Geometry check sheet. Reference: drawing and pictorial views, mm from the part's lowest x, y, z. A direction names the side the tool comes from. Coordinates: 2 decimals unless noted, no trailing zeros. Loops run counter-clockwise (first coordinate to the right, second up) from the corner with the lowest first, then second, coordinate; pieces in that order, holes last. Notation, with made-up numbers: (53, 64.5) -> (91, 64.5) arc R22 cw to (91, 98.5) -> close; hole circle Ø6 at (43.5, -34). An arc over 180 degrees is marked (long way). Answer as a JSON object with one key per item and string values. Group by question number.
Q1. Set-up check for the marked faces 1 and 2: record each of +Z, -Z, +X, -X, +Y, -Y from which the full face is reachable in a straight line by a thin tool's end or side.
Q2. Cross-section at C-C on z = 7. Give the number of separate pieces and of enclosed holes in the cut face, and give its area (3 significant figures).
Q3. Cross-section at B-B on x = 40. Record the boundary of the cut face in (y, z), and give its area (3 significant figures).
Q4. Release check for a two-part mould opening along X. For the marked faces 3, 4 and 5 record: released by +X, released by -X, zero draft, split by the parting line, or undercut.
Q5. Cross-section at D-D on x = 15. Record the boundary of the cut face in (y, z) (1 decimal), and give its area (3 significant figures).
Q6. Gauge pin test, flat ends, axial feed: pin 1 Ø3 at (x, y) = (69.5, 45) entering from -Z; pin 2 Ø8 at (x, y) = (14.5, 39.5) entering from +Z; pin 3 Ø2.5 at (x, y) = (29.83, 12.39) entering from +Z; pin 4 Ø1 at (y, z) = (8, 2) entering from -X. Record the tip position at first contact, or that the pin passes through.
Q7. Cross-section at A-A on y = 40. Record the boundary of the cut face in (x, z).
Q8. Scan lines: L1, parallel to Y at x = 66.5, z = 2.75; L2, parallel to Y at x = 49, z = 6.75 (1 decimal); L3, parallel to Y at x = 12.5, z = 7.25. Record each from-to range of solid material in increasing order.
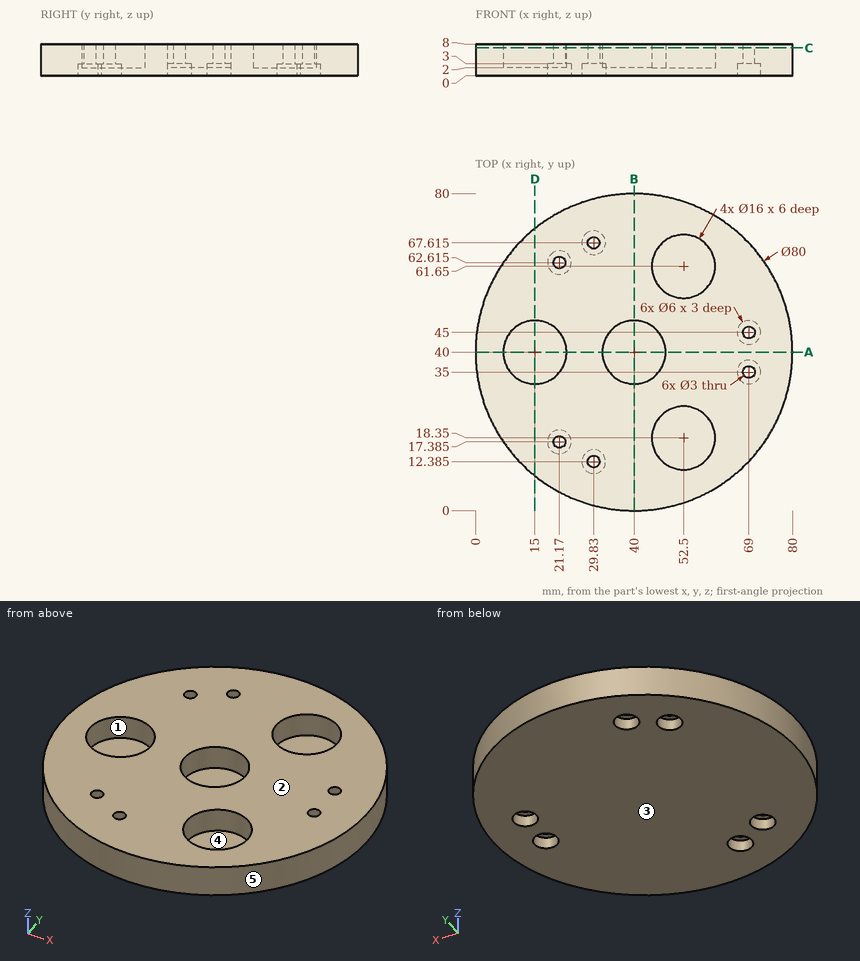
Computed values:
{
 "1": {"face 1": "+Z", "face 2": "+Z, +X, -X, +Y, -Y"},
 "2": {"separate pieces": "1", "enclosed holes": "10", "area": "4,180 mm²"},
 "3": {"outline": "(0, 0) -> (80, 0) -> (80, 8) -> (48, 8) -> (48, 2) -> (32, 2) -> (32, 8) -> (0, 8) -> close", "area": "544 mm²"},
 "4": {"face 3": "zero draft", "face 4": "undercut", "face 5": "split by the parting line"},
 "5": {"outline": "(8.8, 0) -> (71.2, 0) -> (71.2, 8) -> (48, 8) -> (48, 2) -> (32, 2) -> (32, 8) -> (8.8, 8) -> close", "area": "404 mm²"},
 "6": {"pin 1": "stops at z = 3", "pin 2": "stops at z = 2", "pin 3": "passes through", "pin 4": "stops at x = 15.35"},
 "7": {"outline": "(0, 0) -> (80, 0) -> (80, 8) -> (48, 8) -> (48, 2) -> (32, 2) -> (32, 8) -> (23, 8) -> (23, 2) -> (7, 2) -> (7, 8) -> (0, 8) -> close"},
 "8": {"L1": "y = 10.04 to 33.34, 36.66 to 43.34, 46.66 to 69.96", "L2": "y = 1 to 11.2, 25.5 to 54.5, 68.8 to 79", "L3": "y = 10.95 to 32.4, 47.6 to 69.05"}
}
